Source: CAD feature listing. Evaluate the final solid. Frame: model axes, mm. A direction names the side the tool comes from. Coordinates: 2 decimals unless noted, no trailing zeros. Loops run counter-clockwise (first coordinate to the right, second up) from the corner with the lowest first, then second, coordinate; pieces in that order, holes last. Notation, with made-up numbers: (65, 24.25) -> (123, 24.25) arc R16 ccw to (123, 31.25) -> close; hole circle Ø7 at (88.25, 57.5). An arc over 180 degrees is marked (long way). Answer as a JSON object with one key per item and string values. Group by question number.
from build123d import *

# Parameters (mm, degrees)
EXTRUDE_1_DEPTH   = 2
HOLE_WIZARD_M51_D = 5.5
CHAMFER_1_SIZE    = 2


with BuildPart() as part:
    # Эскиз1 → Бобышка-Вытянуть1 (new body)
    with BuildSketch(Plane(origin=(0, 0, 0), x_dir=(1, 0, 0), z_dir=(0, 0, -1))):
        Polygon((0, 0), (0, 60), (40, 60), (40, 40), (20, 40), (20, 0), align=None)
    extrude(amount=EXTRUDE_1_DEPTH)

    # Отверстие с зазором M51 (through all)
    with Locations(Plane(origin=(0, 0, -2), x_dir=(1, 0, 0), z_dir=(0, 0, -1))):
        with Locations((30, 50), (10, 50), (10, 30), (10, 10)):
            Hole(HOLE_WIZARD_M51_D / 2)

    # Фаска1
    chamfer_1_edges = [part.edges().sort_by_distance(p)[0] for p in [
        (0, 0, -1),
        (0, -60, -1),
        (40, -60, -1),
        (40, -40, -1),
        (20, 0, -1),
    ]]
    chamfer(chamfer_1_edges, length=CHAMFER_1_SIZE)


solid = part.part
1. Section query A-A on x = 30. Return loops of the section in (y, z).
2. Mould query, pull axis Y, two halves, no side actions, for faces 3 (the face through (16, -37, 0)), 4 (the face through (39, -59, -1)), 5 (the face through (29, -40, -1)), 6 (the face through (8.52, -32.32, -0.99)). Classes: pulls with the +Y half, pulls with the -Y half, needs draft (parallel to the pull), parting line crosses it, or undercut.
3. Reachability of faces 1 (the face through (20, -21, -1)), 2 (the face through (8.52, -12.32, -0.99)) from +Z, -Z, +X, -X, +Y, -Y: full face, straight path, thin tool, end or side. Return the list, or none.
4. Section query D-D on z = -1.15. Return loops of the section in (x, y), then the cut area to 3 significant figures.
5. Section query B-B on y = -50. Return loops of the section in (x, z).
6. Ray query, L1, parallel to Y at x = 10, z = -1; L2, parallel to X at y = -50, z = -1.2; L3, parallel to X at y = -10, z = -1.2. Return the intervals inside material, ascending.
7. Section query C-C on y = -30. Return loops of the section in (x, z).
8. Pin query (flat end, axial travel): pin 1 Ø4.5 at (x, y) = (10, -10) entering from +Z. Return the tip coordinate at first contact, or that it passes through.
Solved:
{
 "1": {"outline": "(-60, -2) -> (-52.75, -2) -> (-52.75, 0) -> (-60, 0) -> close; (-47.25, -2) -> (-40, -2) -> (-40, 0) -> (-47.25, 0) -> close"},
 "2": {"face 3": "needs draft", "face 4": "pulls with the -Y half", "face 5": "pulls with the +Y half", "face 6": "undercut"},
 "3": {"face 1": "+Z, -Z, +X, +Y", "face 2": "+Z, -Z"},
 "4": {"outline": "(0, -58) -> (2, -60) -> (38, -60) -> (40, -58) -> (40, -42) -> (38, -40) -> (20, -40) -> (20, -2) -> (18, 0) -> (2, 0) -> (0, -2) -> close; hole circle Ø5.5 at (10, -50); hole circle Ø5.5 at (10, -30); hole circle Ø5.5 at (10, -10); hole circle Ø5.5 at (30, -50)", "area": "1,490 mm^2"},
 "5": {"outline": "(0, -2) -> (7.25, -2) -> (7.25, 0) -> (0, 0) -> close; (12.75, -2) -> (27.25, -2) -> (27.25, 0) -> (12.75, 0) -> close; (32.75, -2) -> (40, -2) -> (40, 0) -> (32.75, 0) -> close"},
 "6": {"L1": "-60 to -52.75, -47.25 to -32.75, -27.25 to -12.75, -7.25 to 0", "L2": "0 to 7.25, 12.75 to 27.25, 32.75 to 40", "L3": "0 to 7.25, 12.75 to 20"},
 "7": {"outline": "(0, -2) -> (7.25, -2) -> (7.25, 0) -> (0, 0) -> close; (12.75, -2) -> (20, -2) -> (20, 0) -> (12.75, 0) -> close"},
 "8": {"pin 1": "through"}
}
